CAD build for the part. Positions are in the model's coordinates, mm. Round coordinates to 2 decimals unless told otherwise and drop trailing zeros. Loops run counter-clockwise (first coordinate to the right, second up) from the corner with the lowest first, then second, coordinate; pieces in that order, holes last.
```python
from build123d import *

# Parameters (mm, degrees)
F0_R     = 3.175
F1_DEPTH = 241.3
F4_DEPTH = 6.35
F6_DEPTH = 6.35


with BuildPart() as f1:
    # F0 (on Front) → F1 (new body)
    with BuildSketch(Plane.XZ):
        Circle(F0_R)
    extrude(amount=-F1_DEPTH)

    # F3 (on Right) → F4 (join)
    with BuildSketch(Plane.YZ):
        with BuildLine():
            ThreePointArc((106.045, 0), (109.22, -3.175), (112.395, 0))
            Line((112.395, 0), (106.045, 0))
        make_face()
        with BuildLine():
            Line((106.045, 0), (112.395, 0))
            ThreePointArc((112.395, 0), (109.22, 3.175), (106.045, 0))
        make_face()
    extrude(amount=F4_DEPTH)

    # F5 (on Right) → F6 (join)
    with BuildSketch(Plane.YZ):
        with BuildLine():
            ThreePointArc((136.525, 0), (139.7, -3.175), (142.875, 0))
            Line((142.875, 0), (136.525, 0))
        make_face()
        with BuildLine():
            Line((136.525, 0), (142.875, 0))
            ThreePointArc((142.875, 0), (139.7, 3.175), (136.525, 0))
        make_face()
    extrude(amount=-F6_DEPTH)


solid = f1.part
```
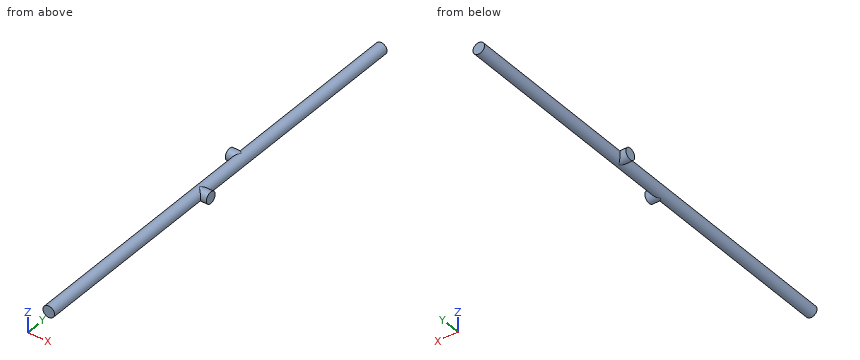
Item 1: Cut at C-C, the plane y = 75. Give the cut face in (x, z) (3 decimals).
Answers follow:
outline: circle Ø6.35 at (0, 0)
Item 2: Cut at A-A, the plane z = 0. Give the cut face in (x, y) (3 decimals), plus the area to 3 significant figures.
Answers follow:
outline: (-6.35, 136.525) - (-3.175, 136.525) - (-3.175, 0) - (3.175, 0) - (3.175, 106.045) - (6.35, 106.045) - (6.35, 112.395) - (3.175, 112.395) - (3.175, 241.3) - (-3.175, 241.3) - (-3.175, 142.875) - (-6.35, 142.875) - close
area: 1,570 mm2
Item 3: Probe line 1 (Z direction, x = -0.25, y = 213); line 2 (Y direction, x = -5.5, z = 0.25); line 3 (Y direction, x = -3.5, z = 0.5). List the from-to ranges inside material, lowest first.
Answers follow:
line 1: z = -3.17 to 3.17
line 2: y = 136.53 to 142.87
line 3: y = 136.56 to 142.84
Item 4: Flat gauge pins, fed straight in: P1, Ø1.5, axis at x = 1, y = 212, coming from the -Z side; P2, Ø1.5, axis at y = 187.5, z = -2.5, coming from the +X side. Where does each tip first touch, or does it go through?
Answers follow:
P1: stops at z = -3.17
P2: stops at x = 2.65
Item 5: Cut at B-B, the plane y = 139.7. Give the cut face in (x, z) (3 decimals), plus the area to 3 significant figures.
Answers follow:
outline: (-6.35, -3.175) - (0, -3.175) arc R3.175 ccw to (0, 3.175) - (-6.35, 3.175) - close
area: 56.2 mm2
